Verification items for the finished model (mm, model axes). Coordinates: 2 decimals unless noted, no trailing zeros. Order: outer loops, then holes, each group sorted by start corner. A loop starts at its lowest first (then second) coordinate and runs counter-clockwise, first axis right, second up. Notation, with made-up numbers: M -21,-36 L -17,-36 A17 ccw -17,-13 Z; hole C 52,55.25 d10. An arc over 180 degrees is marked long. Return JSON: item names as keys, results as strings. Group by question number.
Q1. Section check A-A, the plane y = 0.35. Count the separate pieces of the cut face and the enclosed holes in it, then the cut area to 3 significant figures.
Q2. Mould release check, pull along X, two halves, no side actions. Record for faces 1 (the face through (10.16, 1, 0)), 2 (the face through (0, 1.6, 0)), 3 (the face through (4.87, 0.81, 8.78)): pulls with the +X half, pulls with the -X half, needs draft (parallel to the pull), parting line crosses it, or undercut.
Q3. Thickness scan on probe 1 along Z at (x, y) = (4.5, 0.3); probe 2 along Z at (x, y) = (-0.75, 0.35); probe 3 along X at (y, z) = (1.05, -3.25). Record the ranges inside material, lowest first.
Q4. Section check C-C, the plane z = -4. Enter the section's corners in (x, y).
from build123d import *

# Parameters (mm, degrees)
SKETCH_1_W          = 20.32
SKETCH_1_H          = 21.234
EXTRUDE_1_DEPTH     = 1.6
SKETCH_3_R          = 0.45
CUT_EXTRUDE_1_DEPTH = 15.781958226


with BuildPart() as part:
    # Эскиз1 → Бобышка-Вытянуть1 (new body)
    with BuildSketch(Plane(origin=(0, 0, 0), x_dir=(1, 0, 0), z_dir=(0, 1, 0))):
        Rectangle(SKETCH_1_W, SKETCH_1_H)
    extrude(amount=EXTRUDE_1_DEPTH)

    # Эскиз3 → Вырез-Вытянуть1 (cut, through all)
    with BuildSketch(Plane(origin=(0, 1.6, 0), x_dir=(1, 0, 0), z_dir=(0, 1, 0))):
        with Locations(Location((-8.458, 8.991, 0), (0, 0, 270))):
            Circle(SKETCH_3_R)
        with Locations(Location((-5.918, 8.991, 0), (0, 0, 270))):
            Circle(SKETCH_3_R)
        with Locations(Location((-3.378, 8.991, 0), (0, 0, 270))):
            Circle(SKETCH_3_R)
        with Locations(Location((-0.608, 8.991, 0), (0, 0, 270))):
            Circle(SKETCH_3_R)
        with Locations(Location((1.932, 8.991, 0), (0, 0, 270))):
            Circle(SKETCH_3_R)
        with Locations(Location((4.472, 8.991, 0), (0, 0, 270))):
            Circle(SKETCH_3_R)
        with Locations(Location((4.472, -8.991, 0), (0, 0, 90))):
            Circle(SKETCH_3_R)
        with Locations(Location((1.932, -8.991, 0), (0, 0, 90))):
            Circle(SKETCH_3_R)
        with Locations(Location((-0.608, -8.991, 0), (0, 0, 90))):
            Circle(SKETCH_3_R)
        with Locations(Location((-3.378, -8.991, 0), (0, 0, 90))):
            Circle(SKETCH_3_R)
        with Locations(Location((-5.918, -8.991, 0), (0, 0, 90))):
            Circle(SKETCH_3_R)
        with Locations(Location((-8.458, -8.991, 0), (0, 0, 90))):
            Circle(SKETCH_3_R)
        with Locations(Location((7.239, 8.991, 0), (0, 0, 270))):
            Circle(SKETCH_3_R)
        with Locations(Location((7.239, 6.451, 0), (0, 0, 270))):
            Circle(SKETCH_3_R)
        with Locations(Location((7.239, 3.911, 0), (0, 0, 270))):
            Circle(SKETCH_3_R)
        with Locations(Location((7.239, 1.371, 0), (0, 0, 270))):
            Circle(SKETCH_3_R)
        with Locations(Location((7.239, -1.169, 0), (0, 0, 270))):
            Circle(SKETCH_3_R)
        with Locations(Location((7.239, -3.709, 0), (0, 0, 270))):
            Circle(SKETCH_3_R)
        with Locations(Location((7.239, -6.249, 0), (0, 0, 270))):
            Circle(SKETCH_3_R)
        with Locations(Location((7.239, -8.789, 0), (0, 0, 270))):
            Circle(SKETCH_3_R)
        with Locations(Location((-8.457, 2.875, 0), (0, 0, 270))):
            Circle(SKETCH_3_R)
        with Locations(Location((-8.457, 0.335, 0), (0, 0, 270))):
            Circle(SKETCH_3_R)
        with Locations(Location((-8.457, -2.205, 0), (0, 0, 270))):
            Circle(SKETCH_3_R)
    extrude(amount=-CUT_EXTRUDE_1_DEPTH, mode=Mode.SUBTRACT)


solid = part.part
Numbers:
{
 "1": {"separate pieces": "1", "enclosed holes": "23", "area": "417 mm2"},
 "2": {"face 1": "pulls with the +X half", "face 2": "needs draft", "face 3": "undercut"},
 "3": {"probe 1": "z = -10.62 to -9.44, -8.54 to 8.54, 9.44 to 10.62", "probe 2": "z = -10.62 to -9.42, -8.56 to 8.56, 9.42 to 10.62", "probe 3": "x = -10.16 to -8.71, -8.21 to 10.16"},
 "4": {"outline": "M -10.16,0 L 6.8,0 L 6.8,1.6 L -10.16,1.6 Z; M 7.68,0 L 10.16,0 L 10.16,1.6 L 7.68,1.6 Z"}
}
